```python
from build123d import *

# Parameters (mm, degrees)
F0_W     = 127
F0_H     = 152.4
F0_R     = 6.35
F1_DEPTH = 25.4
F2_W     = 127
F2_H     = 12.7
F3_DEPTH = 381
F4_R     = 31.75
F5_DEPTH = 25.4


with BuildPart() as f1:
    # F0 (on Front) → F1 (new body)
    with BuildSketch(Plane.XZ):
        with Locations((0, 63.5)):
            Rectangle(F0_W, F0_H)
        Circle(F0_R, mode=Mode.SUBTRACT)
    extrude(amount=F1_DEPTH)

    # F2 (on face) → F3 (join)
    with BuildSketch(Plane.XZ.offset(25.4)):
        with Locations((0, 133.35)):
            Rectangle(F2_W, F2_H)
    extrude(amount=F3_DEPTH)

    # F4 (on face) → F5 (cut)
    with BuildSketch(Plane.XY.offset(139.7)):
        with Locations((0, -88.9)):
            Circle(F4_R)
        with Locations((0, -171.45)):
            Circle(F4_R)
        with Locations((0, -254)):
            Circle(F4_R)
        with Locations((0, -336.55)):
            Circle(F4_R)
    extrude(amount=-F5_DEPTH, mode=Mode.SUBTRACT)


solid = f1.part
```
The listing builds one solid part. Answer for the finished solid, in the listing's coordinates (mm). A direction names the side the tool comes from. Round coordinates to 2 decimals unless told otherwise and drop trailing zeros. Write each loop counter-clockwise with the first axis right and the second up, starting at its lowest first coordinate (ties: lowest second). Pieces come first, ordered by that corner, then holes. Notation, with made-up numbers: (-14.5, -17.5) -> (21.5, -17.5) arc R32 cw to (21.5, 8.5) -> close; hole circle Ø7 at (43, -27). An arc over 180 degrees is marked (long way). Answer as a JSON object with one key per item and string values. Group by question number.
Q1. Straight lines are drawn through the part: line 1 along Y through (x, z) = (0, 132); line 2 along Z through (x, y) = (0, -16.75); line 3 along Y through (x, z) = (-38, 30). For each, find the intervals that lie inside material, in ascending order.
Q2. Which of the six approach directions +Z, -Z, +X, -X, +Y, -Y give full straight-line access (tool end or side, diameter ignored) to faces 4 (the face through (-1, -25.4, 58)), 5 (the face through (-63.5, -112, 131))?
Q3. Determine the mould class of faces 1 (the face through (63.5, -112, 131)), 2 (the face through (-6.883, -119.895, 133.439)), 3 (the face through (-1, 0, 65)) for opening direction X: pulls with the +X half, pulls with the -X half, needs draft (parallel to the pull), parting line crosses it, or undercut.
Q4. Section C-C (x = -2) is taken. Write down the section's boundary in (y, z).
Q5. Section B-B (z = 0) is taken. Write down the section's boundary in (x, y).
Q6. Section D-D (z = 16.5) is taken. Write down the section's boundary in (x, y), plus the area to 3 significant figures.
Q7. Section A-A (y = -88.9) is taken. Write down the section's boundary in (x, z), plus the area to 3 significant figures.
Q8. Each of these flat-tipped pins is pushed along its axis until it touches: pin 1 Ø1 at (x, y) = (-43.5, -217) entering from -Z; pin 2 Ø4 at (x, z) = (48, 22) entering from +Y; pin 3 Ø1 at (x, z) = (-36, 4) entering from -Y. Where does it stop, or does it pass through?
Check values:
{
 "1": {"line 1": "-406.4 to -368.3, -304.8 to -285.75, -222.25 to -203.2, -139.7 to -120.65, -57.15 to 0", "line 2": "-12.7 to -6.35, 6.35 to 139.7", "line 3": "-25.4 to 0"},
 "2": {"face 4": "-Z, +X, -X, -Y", "face 5": "+Z, -Z, -X, +Y, -Y"},
 "3": {"face 1": "pulls with the +X half", "face 2": "undercut", "face 3": "needs draft"},
 "4": {"outline": "(-406.4, 127) -> (-368.24, 127) -> (-368.24, 139.7) -> (-406.4, 139.7) -> close; (-304.86, 127) -> (-285.69, 127) -> (-285.69, 139.7) -> (-304.86, 139.7) -> close; (-222.31, 127) -> (-203.14, 127) -> (-203.14, 139.7) -> (-222.31, 139.7) -> close; (-139.76, 127) -> (-120.59, 127) -> (-120.59, 139.7) -> (-139.76, 139.7) -> close; (-57.21, 127) -> (-25.4, 127) -> (-25.4, 6.03) -> (0, 6.03) -> (0, 139.7) -> (-57.21, 139.7) -> close; (-25.4, -12.7) -> (0, -12.7) -> (0, -6.03) -> (-25.4, -6.03) -> close"},
 "5": {"outline": "(-63.5, -25.4) -> (-6.35, -25.4) -> (-6.35, 0) -> (-63.5, 0) -> close; (6.35, -25.4) -> (63.5, -25.4) -> (63.5, 0) -> (6.35, 0) -> close"},
 "6": {"outline": "(-63.5, -25.4) -> (63.5, -25.4) -> (63.5, 0) -> (-63.5, 0) -> close", "area": "3,230 mm^2"},
 "7": {"outline": "(-63.5, 127) -> (-31.75, 127) -> (-31.75, 139.7) -> (-63.5, 139.7) -> close; (31.75, 127) -> (63.5, 127) -> (63.5, 139.7) -> (31.75, 139.7) -> close", "area": "806 mm^2"},
 "8": {"pin 1": "z = 127", "pin 2": "y = 0", "pin 3": "y = -25.4"}
}
